Geometry check sheet. Reference: the model listing, model coordinates, mm. Coordinates: 2 decimals unless noted, no trailing zeros. Write each loop counter-clockwise with the first axis right and the second up, starting at its lowest first coordinate (ties: lowest second). Pieces come first, ordered by that corner, then holes. Notation, with made-up numbers: M 76,72.5 L 100,72.5 A25 ccw 100,105.5 Z; hole C 89.5,83.25 d7. An arc over 180 degrees is marked long. Put each result on its own line as item: value. Start each with the question number.
1) Cross-section at B-B on x = -0.5. Record the cut outline in (y, z), plus the area to 3 significant figures.
2) Scan lines: line 1 along Y through (x, z) = (0, 121.5); line 2 along X through (y, z) = (7.5, 140.5). Record each from-to range of solid material in increasing order.
3) Cross-section at A-A on y = 0. Record the cut outline in (x, z).
4) Gauge pin test, flat ends, axial feed: pin 1 (3.5 mm diameter, centred on y = 0.5, z = 85, fed in from -X); pin 2 (1 mm diameter, centred on x = 2.5, z = 133.5, fed in from -Y); pin 3 (1.3 mm diameter, centred on x = -0.5, z = 41.5, fed in from +Y). Record the tip position at first contact, or that the pin passes through.
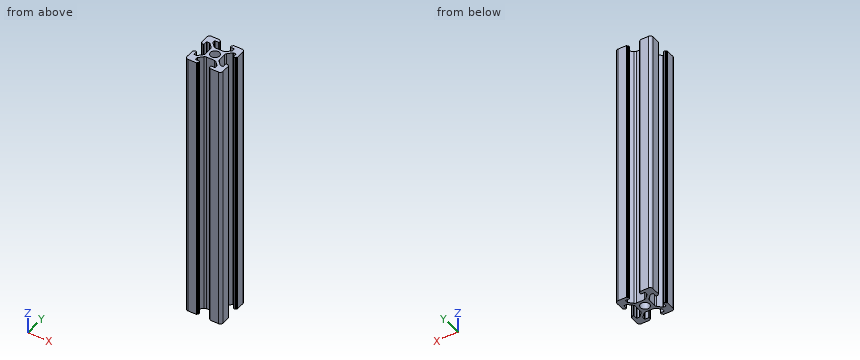
from build123d import *

# Parameters (mm, degrees)
SKETCH_1_R      = 2.5
EXTRUDE_1_DEPTH = 152.4


with BuildPart() as part:
    # 草图1 → 凸台-拉伸1 (new body)
    with BuildSketch(Plane.XY):
        with BuildLine():
            Line((-8.502261885, -10.002261885), (-3.85, -10.002261885))
            ThreePointArc((-3.85, -10.002261885), (-3.673223305, -9.929038581), (-3.6, -9.752261885))
            Line((-3.6, -9.752261885), (-3.6, -9.502261885))
            Line((-3.6, -9.502261885), (-3.35, -9.502261885))
            ThreePointArc((-3.35, -9.502261885), (-3.173223305, -9.429038581), (-3.1, -9.252261885))
            Line((-3.1, -9.252261885), (-3.1, -8.45))
            ThreePointArc((-3.1, -8.45), (-3.173223305, -8.273223305), (-3.35, -8.2))
            Line((-3.35, -8.2), (-5.25, -8.2))
            ThreePointArc((-5.25, -8.2), (-5.426776695, -8.126776695), (-5.5, -7.95))
            Line((-5.5, -7.95), (-5.5, -6.664213562))
            ThreePointArc((-5.5, -6.664213562), (-5.480969883, -6.568542704), (-5.426776695, -6.487436867))
            Line((-5.426776695, -6.487436867), (-3.278679656, -4.339339828))
            ThreePointArc((-3.278679656, -4.339339828), (-2.792044633, -4.014180701), (-2.218019485, -3.9))
            Line((-2.218019485, -3.9), (2.218019485, -3.9))
            ThreePointArc((2.218019485, -3.9), (2.792044633, -4.014180701), (3.278679656, -4.339339828))
            Line((3.278679656, -4.339339828), (5.426776695, -6.487436867))
            ThreePointArc((5.426776695, -6.487436867), (5.480969883, -6.568542704), (5.5, -6.664213562))
            Line((5.5, -6.664213562), (5.5, -7.95))
            ThreePointArc((5.5, -7.95), (5.426776695, -8.126776695), (5.25, -8.2))
            Line((5.25, -8.2), (3.35, -8.2))
            ThreePointArc((3.35, -8.2), (3.173223305, -8.273223305), (3.1, -8.45))
            Line((3.1, -8.45), (3.1, -9.252261885))
            ThreePointArc((3.1, -9.252261885), (3.173223305, -9.429038581), (3.35, -9.502261885))
            Line((3.35, -9.502261885), (3.6, -9.502261885))
            Line((3.6, -9.502261885), (3.6, -9.752261885))
            ThreePointArc((3.6, -9.752261885), (3.673223305, -9.929038581), (3.85, -10.002261885))
            Line((3.85, -10.002261885), (8.502261885, -10.002261885))
            ThreePointArc((8.502261885, -10.002261885), (9.562922057, -9.562922057), (10.002261885, -8.502261885))
            Line((10.002261885, -8.502261885), (10.002261885, -3.85))
            ThreePointArc((10.002261885, -3.85), (9.929038581, -3.673223305), (9.752261885, -3.6))
            Line((9.752261885, -3.6), (9.502261885, -3.6))
            Line((9.502261885, -3.6), (9.502261885, -3.35))
            ThreePointArc((9.502261885, -3.35), (9.429038581, -3.173223305), (9.252261885, -3.1))
            Line((9.252261885, -3.1), (8.45, -3.1))
            ThreePointArc((8.45, -3.1), (8.273223305, -3.173223305), (8.2, -3.35))
            Line((8.2, -3.35), (8.2, -5.25))
            ThreePointArc((8.2, -5.25), (8.126776695, -5.426776695), (7.95, -5.5))
            Line((7.95, -5.5), (6.664213562, -5.5))
            ThreePointArc((6.664213562, -5.5), (6.568542704, -5.480969883), (6.487436867, -5.426776695))
            Line((6.487436867, -5.426776695), (4.339339828, -3.278679656))
            ThreePointArc((4.339339828, -3.278679656), (4.014180701, -2.792044633), (3.9, -2.218019485))
            Line((3.9, -2.218019485), (3.9, 2.218019485))
            ThreePointArc((3.9, 2.218019485), (4.014180701, 2.792044633), (4.339339828, 3.278679656))
            Line((4.339339828, 3.278679656), (6.487436867, 5.426776695))
            ThreePointArc((6.487436867, 5.426776695), (6.568542704, 5.480969883), (6.664213562, 5.5))
            Line((6.664213562, 5.5), (7.95, 5.5))
            ThreePointArc((7.95, 5.5), (8.126776695, 5.426776695), (8.2, 5.25))
            Line((8.2, 5.25), (8.2, 3.35))
            ThreePointArc((8.2, 3.35), (8.273223305, 3.173223305), (8.45, 3.1))
            Line((8.45, 3.1), (9.252261885, 3.1))
            ThreePointArc((9.252261885, 3.1), (9.429038581, 3.173223305), (9.502261885, 3.35))
            Line((9.502261885, 3.35), (9.502261885, 3.6))
            Line((9.502261885, 3.6), (9.752261885, 3.6))
            ThreePointArc((9.752261885, 3.6), (9.929038581, 3.673223305), (10.002261885, 3.85))
            Line((10.002261885, 3.85), (10.002261885, 8.502261885))
            ThreePointArc((10.002261885, 8.502261885), (9.562922057, 9.562922057), (8.502261885, 10.002261885))
            Line((8.502261885, 10.002261885), (3.85, 10.002261885))
            ThreePointArc((3.85, 10.002261885), (3.673223305, 9.929038581), (3.6, 9.752261885))
            Line((3.6, 9.752261885), (3.6, 9.502261885))
            Line((3.6, 9.502261885), (3.35, 9.502261885))
            ThreePointArc((3.35, 9.502261885), (3.173223305, 9.429038581), (3.1, 9.252261885))
            Line((3.1, 9.252261885), (3.1, 8.45))
            ThreePointArc((3.1, 8.45), (3.173223305, 8.273223305), (3.35, 8.2))
            Line((3.35, 8.2), (5.25, 8.2))
            ThreePointArc((5.25, 8.2), (5.426776695, 8.126776695), (5.5, 7.95))
            Line((5.5, 7.95), (5.5, 6.664213562))
            ThreePointArc((5.5, 6.664213562), (5.480969883, 6.568542704), (5.426776695, 6.487436867))
            Line((5.426776695, 6.487436867), (3.278679656, 4.339339828))
            ThreePointArc((3.278679656, 4.339339828), (2.792044633, 4.014180701), (2.218019485, 3.9))
            Line((2.218019485, 3.9), (-2.218019485, 3.9))
            ThreePointArc((-2.218019485, 3.9), (-2.792044633, 4.014180701), (-3.278679656, 4.339339828))
            Line((-3.278679656, 4.339339828), (-5.426776695, 6.487436867))
            ThreePointArc((-5.426776695, 6.487436867), (-5.480969883, 6.568542704), (-5.5, 6.664213562))
            Line((-5.5, 6.664213562), (-5.5, 7.95))
            ThreePointArc((-5.5, 7.95), (-5.426776695, 8.126776695), (-5.25, 8.2))
            Line((-5.25, 8.2), (-3.35, 8.2))
            ThreePointArc((-3.35, 8.2), (-3.173223305, 8.273223305), (-3.1, 8.45))
            Line((-3.1, 8.45), (-3.1, 9.252261885))
            ThreePointArc((-3.1, 9.252261885), (-3.173223305, 9.429038581), (-3.35, 9.502261885))
            Line((-3.35, 9.502261885), (-3.6, 9.502261885))
            Line((-3.6, 9.502261885), (-3.6, 9.752261885))
            ThreePointArc((-3.6, 9.752261885), (-3.673223305, 9.929038581), (-3.85, 10.002261885))
            Line((-3.85, 10.002261885), (-8.502261885, 10.002261885))
            ThreePointArc((-8.502261885, 10.002261885), (-9.562922057, 9.562922057), (-10.002261885, 8.502261885))
            Line((-10.002261885, 8.502261885), (-10.002261885, 3.85))
            ThreePointArc((-10.002261885, 3.85), (-9.929038581, 3.673223305), (-9.752261885, 3.6))
            Line((-9.752261885, 3.6), (-9.502261885, 3.6))
            Line((-9.502261885, 3.6), (-9.502261885, 3.35))
            ThreePointArc((-9.502261885, 3.35), (-9.429038581, 3.173223305), (-9.252261885, 3.1))
            Line((-9.252261885, 3.1), (-8.45, 3.1))
            ThreePointArc((-8.45, 3.1), (-8.273223305, 3.173223305), (-8.2, 3.35))
            Line((-8.2, 3.35), (-8.2, 5.25))
            ThreePointArc((-8.2, 5.25), (-8.126776695, 5.426776695), (-7.95, 5.5))
            Line((-7.95, 5.5), (-6.664213562, 5.5))
            ThreePointArc((-6.664213562, 5.5), (-6.568542704, 5.480969883), (-6.487436867, 5.426776695))
            Line((-6.487436867, 5.426776695), (-4.339339828, 3.278679656))
            ThreePointArc((-4.339339828, 3.278679656), (-4.014180701, 2.792044633), (-3.9, 2.218019485))
            Line((-3.9, 2.218019485), (-3.9, -2.218019485))
            ThreePointArc((-3.9, -2.218019485), (-4.014180701, -2.792044633), (-4.339339828, -3.278679656))
            Line((-4.339339828, -3.278679656), (-6.487436867, -5.426776695))
            ThreePointArc((-6.487436867, -5.426776695), (-6.568542704, -5.480969883), (-6.664213562, -5.5))
            Line((-6.664213562, -5.5), (-7.95, -5.5))
            ThreePointArc((-7.95, -5.5), (-8.126776695, -5.426776695), (-8.2, -5.25))
            Line((-8.2, -5.25), (-8.2, -3.35))
            ThreePointArc((-8.2, -3.35), (-8.273223305, -3.173223305), (-8.45, -3.1))
            Line((-8.45, -3.1), (-9.252261885, -3.1))
            ThreePointArc((-9.252261885, -3.1), (-9.429038581, -3.173223305), (-9.502261885, -3.35))
            Line((-9.502261885, -3.35), (-9.502261885, -3.6))
            Line((-9.502261885, -3.6), (-9.752261885, -3.6))
            ThreePointArc((-9.752261885, -3.6), (-9.929038581, -3.673223305), (-10.002261885, -3.85))
            Line((-10.002261885, -3.85), (-10.002261885, -8.502261885))
            ThreePointArc((-10.002261885, -8.502261885), (-9.562922057, -9.562922057), (-8.502261885, -10.002261885))
        make_face()
        Circle(SKETCH_1_R, mode=Mode.SUBTRACT)
    extrude(amount=EXTRUDE_1_DEPTH)


solid = part.part
Answer key:
1. outline: M -3.9,0 L -2.45,0 L -2.45,152.4 L -3.9,152.4 Z; M 2.45,0 L 3.9,0 L 3.9,152.4 L 2.45,152.4 Z
1. area: 442 mm²
2. line 1: y = -3.9 to -2.5, 2.5 to 3.9
2. line 2: x = -10 to -5.5, 5.5 to 10
3. outline: M -3.9,0 L -2.5,0 L -2.5,152.4 L -3.9,152.4 Z; M 2.5,0 L 3.9,0 L 3.9,152.4 L 2.5,152.4 Z
4. pin 1: stops at x = -3.9
4. pin 2: stops at y = -4.12
4. pin 3: stops at y = 3.9
